Work out the finished part from the listing and answer in its coordinate system (mm). A direction names the side the tool comes from. Round coordinates to 2 decimals unless told otherwise and drop trailing zeros. Order: outer loops, then holes, each group sorted by start corner. A loop starts at its lowest first (then second) coordinate and runs counter-clockwise, first axis right, second up. Notation, with made-up numbers: M 51.5,-22 L 76.5,-22 A26 ccw 76.5,14 Z; hole C -19.75,6.5 d8. An arc over 180 degrees is marked long. Return JSON: item names as keys, results as strings.
from build123d import *


# Not quite as in the source:
# - a feature names something its author has since deleted; it is built from what else it names


with BuildPart() as f1:
    # F0 (on Front) → F1 (revolve)
    with BuildSketch(Plane.XZ):
        with BuildLine():
            Line((-55, 60), (-41, 60))
            ThreePointArc((-41, 60), (-40.2928932188, 59.7071067812), (-40, 59))
            Line((-40, 59), (-40, 29.71056928))
            ThreePointArc((-40, 29.71056928), (-39.9785413088, 29.5045185412), (-39.9150861861, 29.3073109607))
            Line((-39.9150861861, 29.3073109607), (-27, 0))
            Line((-27, 0), (-25, 0))
            Line((-25, 0), (-37.9150861861, 29.3073109607))
            ThreePointArc((-37.9150861861, 29.3073109607), (-37.9785413088, 29.5045185412), (-38, 29.71056928))
            Line((-38, 29.71056928), (-38, 59.5))
            ThreePointArc((-38, 59.5), (-38.2928932188, 60.2071067812), (-39, 60.5))
            Line((-39, 60.5), (-55, 60.5))
            Line((-55, 60.5), (-55, 60))
        make_face()
    revolve(axis=Axis((0, 0, 19.5262523685), (0, 0, 1)))


solid = f1.part
Item 1: Find section C-C (z = 37). Determine the outline of the cut face in (x, y).
Output:
{"outline": "C 0,0 d80; hole C 0,0 d76"}
Item 2: Find section D-D (z = 11). Determine the outline of the cut face in (x, y), plus the area to 3 significant figures.
Output:
{"outline": "C 0,0 d63.69; hole C 0,0 d59.69", "area": "388 mm^2"}
Item 3: Which of the six approach directions +Z, -Z, +X, -X, +Y, -Y give full straight-line access (tool end or side, diameter ignored) to faces 1 (the conical face through (-11.909, 22.896, 1.833)), 2 (the cylindrical face through (8.67, 39.05, 44.15))?
Output:
{"face 1": "+Z", "face 2": "-Z"}
Item 4: Each of these flat-tipped pins is pushed along its axis until it touches: pin 1 (10 mm diameter, centred on x = 37, z = 35.5, fed in from +Y); pin 2 (6 mm diameter, centred on y = 14.5, z = 20.5, fed in from +X); pin 3 (10 mm diameter, centred on y = -27.5, z = 40.5, fed in from -X). Where does it stop, or does it pass through?
Output:
{"pin 1": "stops at y = 24", "pin 2": "stops at x = 34.85", "pin 3": "stops at x = -33.07"}
Item 5: Consider line 1 along X through (y, z) = (0, 51.5); line 2 along X through (y, z) = (2, 40). Determine where each line is inside the solid, lowest interval first. Write a range as [from, to].
Output:
{"line 1": "x = [-40, -38], [38, 40]", "line 2": "x = [-39.95, -37.95], [37.95, 39.95]"}
Item 6: The mould has two halves that part along X. Classify faces 3 (the cylindrical face through (-17.535, 33.713, 44.814)), 4 (the flat face through (41, 4, 60)), 5 (the cylindrical face through (11.923, 53.692, 60.246)): pulls with the +X half, pulls with the -X half, needs draft (parallel to the pull), parting line crosses it, or undercut.
Output:
{"face 3": "undercut", "face 4": "needs draft", "face 5": "parting line crosses it"}
Item 7: Find section A-A (y = 0). Determine the outline of the cut face in (x, z).
Output:
{"outline": "M -55,60 L -41,60 A1 cw -40,59 L -40,29.71 A1 ccw -39.92,29.31 L -27,0 L -25,0 L -37.92,29.31 A1 cw -38,29.71 L -38,59.5 A1 ccw -39,60.5 L -55,60.5 Z; M 25,0 L 27,0 L 39.92,29.31 A1 ccw 40,29.71 L 40,59 A1 cw 41,60 L 55,60 L 55,60.5 L 39,60.5 A1 ccw 38,59.5 L 38,29.71 A1 cw 37.92,29.31 Z"}
